Can you work these out from the model? Positions are in its coordinate system, mm. A direction names the side the tool comes from. Give positions to 0.01 mm unless a question says otherwise; leave off trailing zeros. Write each loop counter-clockwise with the first axis right and the second up, starting at its lowest first coordinate (ties: lowest second). Pieces come first, ordered by that corner, then holes. Notation, with made-up numbers: (48, 41) -> (89, 41) arc R14 cw to (89, 56) -> close; hole circle Ø6 at (49, 56.25). An arc over 180 degrees is marked (long way). One line per item, written item: value.
from build123d import *

# Parameters (mm, degrees)
F1_DEPTH = 25.4
F2_W     = 10.3401243687
F2_H     = 10.7896951959
F3_DEPTH = 2.54
F4_W     = 10.3547675535
F4_H     = 10.7866246253
F5_DEPTH = 2.54


with BuildPart() as f1:
    # F0 (on Top) → F1 (new body)
    with BuildSketch(Plane.XY):
        with BuildLine():
            ThreePointArc((33.1865631623, 19.1602711752), (37.0148015337, 9.918086179), (38.3205423505, 0))
            ThreePointArc((38.3205423505, 0), (37.0148015337, -9.918086179), (33.1865631623, -19.1602711752))
            ThreePointArc((33.1865631623, -19.1602711752), (52.3468343375, -14.0262919871), (66.3731263246, 0))
            ThreePointArc((66.3731263246, 0), (52.3468343375, 14.0262919871), (33.1865631623, 19.1602711752))
        make_face()
        with BuildLine():
            ThreePointArc((0, 38.3205423505), (19.1602711752, 33.1865631623), (33.1865631623, 19.1602711752))
            ThreePointArc((33.1865631623, 19.1602711752), (37.0148015337, 28.4024561715), (38.3205423505, 38.3205423505))
            ThreePointArc((38.3205423505, 38.3205423505), (37.0148015337, 48.2386285294), (33.1865631623, 57.4808135257))
            ThreePointArc((33.1865631623, 57.4808135257), (14.0262919871, 52.3468343375), (0, 38.3205423505))
        make_face()
        with BuildLine():
            ThreePointArc((38.3205423505, 38.3205423505), (37.0148015337, 28.4024561715), (33.1865631623, 19.1602711752))
            ThreePointArc((33.1865631623, 19.1602711752), (52.3468343375, 14.0262919871), (66.3731263246, 0))
            ThreePointArc((66.3731263246, 0), (70.201364696, 9.2421849963), (71.5071055127, 19.1602711752))
            ThreePointArc((71.5071055127, 19.1602711752), (60.283278517, 46.25698653), (33.1865631623, 57.4808135257))
            ThreePointArc((33.1865631623, 57.4808135257), (37.0148015337, 48.2386285294), (38.3205423505, 38.3205423505))
        make_face()
        with BuildLine():
            ThreePointArc((38.3205423505, -38.3205423505), (37.0148015337, -28.4024561715), (33.1865631623, -19.1602711752))
            ThreePointArc((33.1865631623, -19.1602711752), (19.1602711752, -33.1865631623), (0, -38.3205423505))
            ThreePointArc((0, -38.3205423505), (14.0262919871, -52.3468343375), (33.1865631623, -57.4808135257))
            ThreePointArc((33.1865631623, -57.4808135257), (37.0148015337, -48.2386285294), (38.3205423505, -38.3205423505))
        make_face()
        with BuildLine():
            ThreePointArc((66.3731263246, 0), (52.3468343375, -14.0262919871), (33.1865631623, -19.1602711752))
            ThreePointArc((33.1865631623, -19.1602711752), (37.0148015337, -28.4024561715), (38.3205423505, -38.3205423505))
            ThreePointArc((38.3205423505, -38.3205423505), (37.0148015337, -48.2386285294), (33.1865631623, -57.4808135257))
            ThreePointArc((33.1865631623, -57.4808135257), (60.283278517, -46.25698653), (71.5071055127, -19.1602711752))
            ThreePointArc((71.5071055127, -19.1602711752), (70.201364696, -9.2421849963), (66.3731263246, 0))
        make_face()
        with BuildLine():
            ThreePointArc((-33.1865631623, 57.4808135257), (-14.0262919871, 52.3468343375), (0, 38.3205423505))
            ThreePointArc((0, 38.3205423505), (14.0262919871, 52.3468343375), (33.1865631623, 57.4808135257))
            ThreePointArc((33.1865631623, 57.4808135257), (0, 76.6410847009), (-33.1865631623, 57.4808135257))
        make_face()
        with BuildLine():
            ThreePointArc((-33.1865631623, 19.1602711752), (-19.1602711752, 33.1865631623), (0, 38.3205423505))
            ThreePointArc((0, 38.3205423505), (-14.0262919871, 52.3468343375), (-33.1865631623, 57.4808135257))
            ThreePointArc((-33.1865631623, 57.4808135257), (-38.3205423505, 38.3205423505), (-33.1865631623, 19.1602711752))
        make_face()
        with BuildLine():
            ThreePointArc((-33.1865631623, -57.4808135257), (-14.0262919871, -52.3468343375), (0, -38.3205423505))
            ThreePointArc((0, -38.3205423505), (-19.1602711752, -33.1865631623), (-33.1865631623, -19.1602711752))
            ThreePointArc((-33.1865631623, -19.1602711752), (-38.3205423505, -38.3205423505), (-33.1865631623, -57.4808135257))
        make_face()
        with BuildLine():
            ThreePointArc((33.1865631623, -57.4808135257), (14.0262919871, -52.3468343375), (0, -38.3205423505))
            ThreePointArc((0, -38.3205423505), (-14.0262919871, -52.3468343375), (-33.1865631623, -57.4808135257))
            ThreePointArc((-33.1865631623, -57.4808135257), (0, -76.6410847009), (33.1865631623, -57.4808135257))
        make_face()
        with BuildLine():
            ThreePointArc((-66.3731263246, 0), (-52.3468343375, 14.0262919871), (-33.1865631623, 19.1602711752))
            ThreePointArc((-33.1865631623, 19.1602711752), (-38.3205423505, 38.3205423505), (-33.1865631623, 57.4808135257))
            ThreePointArc((-33.1865631623, 57.4808135257), (-66.3731263246, 38.3205423505), (-66.3731263246, 0))
        make_face()
        with BuildLine():
            ThreePointArc((-33.1865631623, -19.1602711752), (-38.3205423505, 0), (-33.1865631623, 19.1602711752))
            ThreePointArc((-33.1865631623, 19.1602711752), (-52.3468343375, 14.0262919871), (-66.3731263246, 0))
            ThreePointArc((-66.3731263246, 0), (-52.3468343375, -14.0262919871), (-33.1865631623, -19.1602711752))
        make_face()
        with BuildLine():
            ThreePointArc((-33.1865631623, -57.4808135257), (-38.3205423505, -38.3205423505), (-33.1865631623, -19.1602711752))
            ThreePointArc((-33.1865631623, -19.1602711752), (-52.3468343375, -14.0262919871), (-66.3731263246, 0))
            ThreePointArc((-66.3731263246, 0), (-66.3731263246, -38.3205423505), (-33.1865631623, -57.4808135257))
        make_face()
    extrude(amount=F1_DEPTH)

    # F2 (on face) → F3 (join)
    with BuildSketch(Plane.XY.offset(25.4)):
        with Locations((-5.1700621843, -5.3948475979)):
            Rectangle(F2_W, F2_H)
        with Locations((-5.1700621843, 5.3948475979)):
            Rectangle(F2_W, F2_H)
        with Locations((5.1700621843, 5.3948475979)):
            Rectangle(F2_W, F2_H)
        with Locations((5.1700621843, -5.3948475979)):
            Rectangle(F2_W, F2_H)
        Polygon((-38.5132133961, 0), (-10.3401243687, 0), (-10.3401243687, 10.7896951959), (0, 10.7896951959), (0, 38.3205423505), (-38.5132133961, 38.3205423505), align=None)
        Polygon((38.3205423505, 0), (10.3401243687, 0), (10.3401243687, -10.7896951959), (0, -10.7896951959), (0, -38.3205423505), (38.3205423505, -38.3205423505), align=None)
    extrude(amount=F3_DEPTH)

    # F4 (on face) → F5 (join)
    with BuildSketch(Plane(origin=(0, 0, 0), x_dir=(1, 0, 0), z_dir=(0, 0, -1))):
        Polygon((0, 10.7866246253), (0, 38.3205423505), (-38.3205423505, 38.3205423505), (-38.3205423505, 0), (-10.3547675535, 0), (-10.3547675535, 10.7866246253), align=None)
        with Locations((5.1773837768, 5.3933123127)):
            Rectangle(F4_W, F4_H)
        with Locations((-5.1773837768, 5.3933123127)):
            Rectangle(F4_W, F4_H)
        with Locations((-5.1773837768, -5.3933123127)):
            Rectangle(F4_W, F4_H)
        with Locations((5.1773837768, -5.3933123127)):
            Rectangle(F4_W, F4_H)
        Polygon((38.3205423505, 0), (10.3547675535, 0), (10.3547675535, -10.7866246253), (0, -10.7866246253), (0, -38.3205423505), (38.3205423505, -38.3205423505), align=None)
    extrude(amount=F5_DEPTH)


solid = f1.part
1) We'd pull the mould along Z, two halves only. Please class faces 3 (the face through (-1, 1, 27.94)), 4 (the face through (-66.089, 38.805, 12.522)), 5 (the face through (-1, -1, -2.54)), 6 (the face through (-1, 1, 25.4)): released by +Z, released by -Z, zero draft, split by the parting line, or undercut.
Answer list:
face 3: released by +Z
face 4: zero draft
face 5: released by -Z
face 6: undercut
2) If we section it at A-A (x = 14.5): Write out the boundary of the cut face in (y, z), and give its area (3 significant figures).
Answer list:
outline: (-73.79, 0) -> (-35.47, 0) -> (-35.47, 25.4) -> (0, 25.4) -> (0, 27.94) -> (-38.32, 27.94) -> (-38.32, 25.4) -> (-73.79, 25.4) -> close; (0, -2.54) -> (38.32, -2.54) -> (38.32, 0) -> (73.79, 0) -> (73.79, 25.4) -> (35.47, 25.4) -> (35.47, 0) -> (0, 0) -> close
area: 2,140 mm^2
3) I need wall thicknesses on L1, parallel to Z at x = 0.5, y = -9; L2, parallel to Z at x = -23, y = -48; L3, parallel to Y at x = -19.5, z = 12. Which ranges of each line are inside material? Lowest first, please.
Answer list:
L1: z = -2.54 to 0, 25.4 to 27.94
L2: z = 0 to 25.4
L3: y = -71.31 to -32.99, 32.99 to 71.31
4) For faces 1 (the face through (-1, -1, 0)), 2 (the face through (0.562, 76.637, 12.522)), which set-ups out of +Z, -Z, +X, -X, +Y, -Y let a thin tool reach every point of the face, with its end or its side?
Answer list:
face 1: none
face 2: +Z, -Z, +Y
5) Will these pins go through, and if not, where does the flat tip stop? pin 1 (2 mm diameter, centred on x = 10.5, z = 26, fed in from -Y); pin 2 (2 mm diameter, centred on x = 5, z = -1.5, fed in from -Y); pin 3 (3 mm diameter, centred on x = -22, z = 17.5, fed in from +Y).
Answer list:
pin 1: stops at y = -75.39
pin 2: stops at y = -10.79
pin 3: stops at y = 70.7
6) If we section it at C-C (z = 6.5): Write out the boundary of the cut face in (x, y).
Answer list:
outline: (-66.37, 0) arc R38.32 ccw to (-33.19, -57.48) arc R38.32 ccw to (33.19, -57.48) arc R38.32 ccw to (66.37, 0) arc R38.32 ccw to (33.19, 57.48) arc R38.32 ccw to (-33.19, 57.48) arc R38.32 ccw to start; hole circle Ø76.64 at (0, 0)
7) If we section it at D-D (x = -53): Write out the boundary of the cut face in (y, z).
Answer list:
outline: (-51.96, 0) -> (51.96, 0) -> (51.96, 25.4) -> (-51.96, 25.4) -> close
8) If we section it at B-B (y = -27): Write out the boundary of the cut face in (x, z), and give its area (3 significant figures).
Answer list:
outline: (-70.7, 0) -> (-38.32, 0) -> (-38.32, -2.54) -> (0, -2.54) -> (0, 0) -> (-27.19, 0) -> (-27.19, 25.4) -> (-70.7, 25.4) -> close; (0, 25.4) -> (27.19, 25.4) -> (27.19, 0) -> (70.7, 0) -> (70.7, 25.4) -> (38.32, 25.4) -> (38.32, 27.94) -> (0, 27.94) -> close
area: 2,400 mm^2
